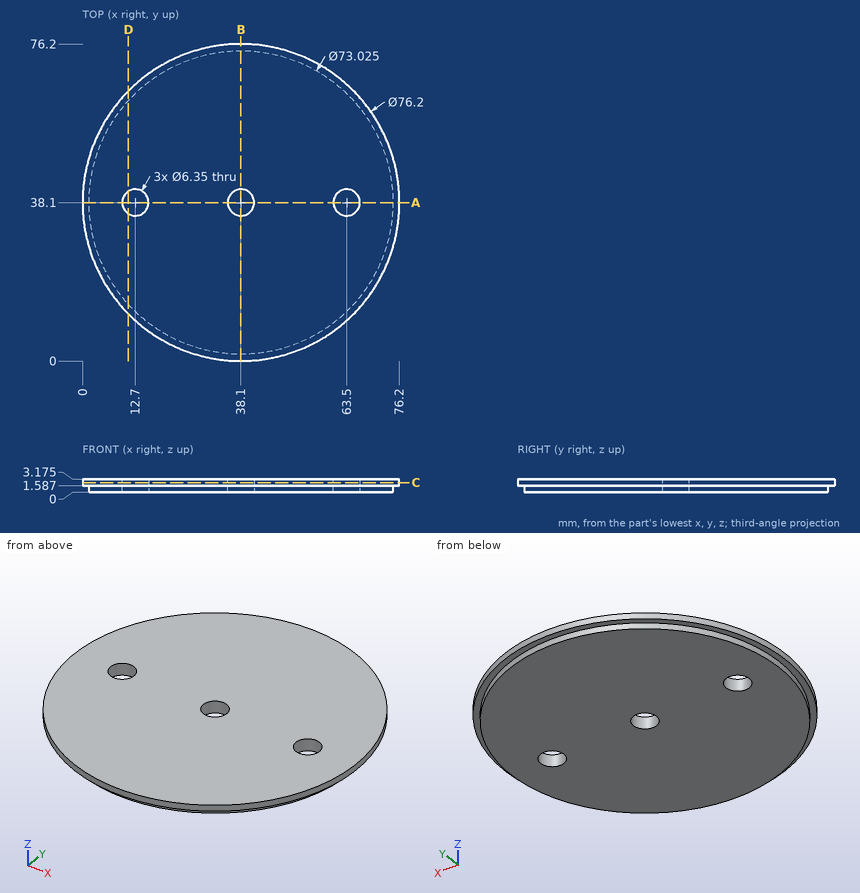
Verification items for this drawing (mm, ordinates from the low corner). Coordinates: 2 decimals unless noted, no trailing zeros. Loops run counter-clockwise (first coordinate to the right, second up) from the corner with the lowest first, then second, coordinate; pieces in that order, holes last. Notation, with made-up numbers: (56, -13.5) - (97, -13.5) arc R28 cw to (97, 13.5) - close; hole circle Ø11 at (88, 67.5). An arc over 180 degrees is marked (long way). One line per item, written item: value. Start each with the question number.
(1) Material ranges on line 1 (Y direction, x = 38.1, z = 1.9) (1 decimal); line 2 (Z direction, x = 21, y = 5.5) (1 decimal); line 3 (Y direction, x = 14, z = 1) (1 decimal), recorded low to high. Write a range as [from, to].
(2) Cross-section at B-B on x = 38.1. Enter the section's corners in (y, z) (1 decimal), plus the area to 3 significant figures.
(3) Cross-section at D-D on x = 11. Enter the section's corners in (y, z) (1 decimal).
(4) Depth check by flat-ended pin: P1, Ø1.5, axis at y = 13.5, z = 0.5, coming from the +X side (1 decimal). Enter the tip coordinate at first touch or a pass-through.
(5) Cross-section at A-A on y = 38.1. Enter the section's corners in (x, z) (1 decimal).
(6) Cross-section at C-C on z = 2.3. Count the separate pieces of the cut face and the enclosed holes in it, plus the area to 3 significant figures.
Results below:
1. line 1: y = [0, 34.9], [41.3, 76.2]
1. line 2: z = [1.6, 3.2]
1. line 3: y = [10.7, 35.2], [41, 65.5]
2. outline: (0, 1.6) - (1.6, 1.6) - (1.6, 0) - (34.9, 0) - (34.9, 3.2) - (0, 3.2) - close; (41.3, 0) - (74.6, 0) - (74.6, 1.6) - (76.2, 1.6) - (76.2, 3.2) - (41.3, 3.2) - close
2. area: 217 mm2
3. outline: (11.3, 1.6) - (13.6, 1.6) - (13.6, 0) - (35.4, 0) - (35.4, 3.2) - (11.3, 3.2) - close; (40.8, 0) - (62.6, 0) - (62.6, 1.6) - (64.9, 1.6) - (64.9, 3.2) - (40.8, 3.2) - close
4. P1: stops at x = 65.7
5. outline: (0, 1.6) - (1.6, 1.6) - (1.6, 0) - (9.5, 0) - (9.5, 3.2) - (0, 3.2) - close; (15.9, 0) - (34.9, 0) - (34.9, 3.2) - (15.9, 3.2) - close; (41.3, 0) - (60.3, 0) - (60.3, 3.2) - (41.3, 3.2) - close; (66.7, 0) - (74.6, 0) - (74.6, 1.6) - (76.2, 1.6) - (76.2, 3.2) - (66.7, 3.2) - close
6. separate pieces: 1
6. enclosed holes: 3
6. area: 4,470 mm2
